from build123d import *

# Parameters (mm, degrees)
EXTRUDE_THIN1_DEPTH = 60
SKETCH2_R           = 4
SKETCH2_R_2         = 2
EXTRUDE_THIN2_DEPTH = 60


with BuildPart() as part:
    # Sketch1 → Extrude-Thin1 (new body)
    with BuildSketch(Plane(origin=(0, 0, 0), x_dir=(1, 0, 0), z_dir=(0, 1, 0))):
        Polygon((3.624997168, -3.44374731), (4.794871238, 1.417465981), (1.16987407, 4.861213291), (-3.624997168, 3.44374731), (-4.794871238, -1.417465981), (-1.16987407, -4.861213291), align=None)
        Polygon((1.950682695, -1.853148561), (2.580215078, 0.762766489), (0.629532383, 2.615915049), (-1.950682695, 1.853148561), (-2.580215078, -0.762766489), (-0.629532383, -2.615915049), align=None, mode=Mode.SUBTRACT)
    extrude(amount=EXTRUDE_THIN1_DEPTH)

    # Sketch2 → Extrude-Thin2 (add)
    with BuildSketch(Plane(origin=(0, 60, 0), x_dir=(1, 0, 0), z_dir=(0, 1, 0))):
        Circle(SKETCH2_R)
        Circle(SKETCH2_R_2, mode=Mode.SUBTRACT)
    extrude(amount=-EXTRUDE_THIN2_DEPTH)


solid = part.part
Can you work these out from the model? Positions are in its coordinate system, mm. Coordinates: 2 decimals unless noted, no trailing zeros. Loops run counter-clockwise (first coordinate to the right, second up) from the corner with the lowest first, then second, coordinate; pieces in that order, holes last. Notation, with made-up numbers: (-9.75, 7) - (49.25, 7) arc R22 ccw to (49.25, 32) - close; hole circle Ø9 at (4.5, 78.5). An arc over 180 degrees is marked (long way). Answer as a JSON object with one key per item and string values. Group by question number.
Item 1: If we section it at B-B (x = 0): List the corners of the cut face in (y, z) for me, plus the area to 3 significant figures.
Item 2: If I drill on L1, parallel to Z at x = -0.5, y = 22; L2, parallel to Z at x = -1.5, y = 38; L3, parallel to X at y = 24, z = 0, over which ranges is the centre line in solid material (lowest first)? Write a range as from..to.
Item 3: If we section it at A-A (y = 55.5): List the corners of the cut face in (x, z) for me (3 decimals), plus the area to 3 significant figures.
Item 4: If we mould it in two halves opening along Z, with no side actions, what happens to faces 1 (the face through (3.008, 29.58, -3.115)), 2 (the face through (-0.1, 0, -2.2)), 3 (the face through (0, 30, 2)), 4 (the face through (1.194, 29.58, 4.162))? For each: released by +Z, released by -Z, zero draft, split by the parting line, or undercut.
Item 5: If we section it at D-D (z = 2.75): List the corners of the cut face in (x, y) for me, plus the area to 3 significant figures.
Item 6: For pin 1 (5 mm diameter, centred on y = 42.5, z = -4, fed in from +X); pin 2 (3 mm diameter, centred on x = -2, z = -2.5, fed in from -Y); pin 3 (2 mm diameter, centred on y = 33, z = -0.5, fed in from -X); pin 4 (2 mm diameter, centred on x = 0.5, y = 44.5, fed in from +Z), each with a flat end and sliding along its axis, tell me the tip position at first contact or that it passes through.
Item 7: If we section it at C-C (z = -0.5): List the corners of the cut face in (x, y) for me.
Returned:
{
 "1": {"outline": "(0, -4.52) - (60, -4.52) - (60, -2) - (0, -2) - close; (0, 2) - (60, 2) - (60, 4.52) - (0, 4.52) - close", "area": "302 mm²"},
 "2": {"L1": "z = -4.37..-1.94, 1.94..4.66", "L2": "z = -4.07..-1.32, 1.32..4.55", "L3": "x = -4.45..-2, 2..4.45"},
 "3": {"outline": "(-4.795, 1.417) - (-3.625, -3.444) - (1.17, -4.861) - (4.795, -1.417) - (3.625, 3.444) - (-1.17, 4.861) - close; hole circle Ø4 at (0, 0)", "area": "52.4 mm²"},
 "4": {"face 1": "released by -Z", "face 2": "zero draft", "face 3": "undercut", "face 4": "released by +Z"},
 "5": {"outline": "(-3.39, 0) - (3.79, 0) - (3.79, 60) - (-3.39, 60) - close", "area": "431 mm²"},
 "6": {"pin 1": "stops at x = 4.71", "pin 2": "stops at y = 0", "pin 3": "stops at x = -4.57", "pin 4": "stops at z = 4.66"},
 "7": {"outline": "(-4.33, 0) - (-1.94, 0) - (-1.94, 60) - (-4.33, 60) - close; (1.94, 0) - (4.57, 0) - (4.57, 60) - (1.94, 60) - close"}
}
